```python
from build123d import *

# Parameters (mm, degrees)
F1_DEPTH = 7.5


with BuildPart() as f1:
    # F0 (on Top) → F1 (new body)
    with BuildSketch(Plane.XY):
        with BuildLine():
            ThreePointArc((0, 2), (0.585786, 0.585786), (2, 0))
            Line((2, 0), (8, 0))
            ThreePointArc((8, 0), (9.414214, 0.585786), (10, 2))
            Line((10, 2), (10, 45))
            ThreePointArc((10, 45), (9.414214, 46.414214), (8, 47))
            Line((8, 47), (-8.8, 47))
            ThreePointArc((-8.8, 47), (-10.214214, 46.414214), (-10.8, 45))
            Line((-10.8, 45), (-10.8, 39))
            ThreePointArc((-10.8, 39), (-10.214214, 37.585786), (-8.8, 37))
            Line((-8.8, 37), (-7.8, 37))
            ThreePointArc((-7.8, 37), (-6.385786, 37.585786), (-5.8, 39))
            Line((-5.8, 39), (-5.8, 42))
            Line((-5.8, 42), (0, 42))
            Line((0, 42), (0, 2))
        make_face()
    extrude(amount=F1_DEPTH)


solid = f1.part
```
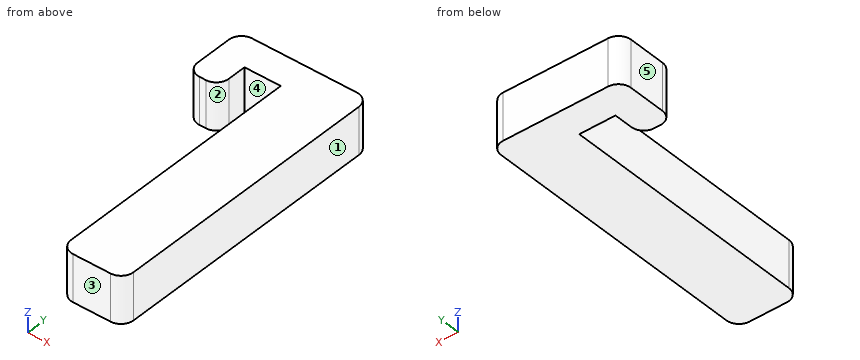
Geometry check sheet. Reference: the model listing, model coordinates, mm. Face numbers are marked on the shaded views. A direction names the side the tool comes from. Give positions to 0.01 mm unless a question says otherwise; leave off trailing zeros. Write each loop counter-clockwise with the first axis right and the second up, starting at its lowest first coordinate (ties: lowest second). Pieces come first, ordered by that corner, then holes. Notation, with made-up numbers: (-27.5, 36) - (17.5, 36) arc R30 ccw to (17.5, 67) - close; hole circle Ø7 at (54, -4.75). An arc over 180 degrees is marked (long way). Use a Markdown table: item, result.
Q1. Section check C-C, the plane x = -0.5. Enter the section's corners in (y, z).
Computed:
| item | result |
|---|---|
| outline | (42, 0) - (47, 0) - (47, 7.5) - (42, 7.5) - close |
Q2. Section check D-D, the plane y = 19. Enter the section's corners in (x, z).
Computed:
| item | result |
|---|---|
| outline | (0, 0) - (10, 0) - (10, 7.5) - (0, 7.5) - close |
Q3. Section check A-A, the plane y = 41. Enter the section's corners in (x, z), then the cut area to 4 significant figures.
Computed:
| item | result |
|---|---|
| outline | (-10.8, 0) - (-5.8, 0) - (-5.8, 7.5) - (-10.8, 7.5) - close; (0, 0) - (10, 0) - (10, 7.5) - (0, 7.5) - close |
| area | 112.5 mm² |
Q4. Set-up check for the marked faces 4 and 5: record each of +Z, -Z, +X, -X, +Y, -Y from which the full face is reachable in a straight line by a thin tool's end or side.
Computed:
| item | result |
|---|---|
| face 4 | +Z, -Z, -Y |
| face 5 | +Z, -Z, -X, +Y, -Y |
Q5. Thickness scan on L1, parallel to X at y = 19.5, z = 7; L2, parallel to Y at x = -8.5, z = 2; L3, parallel to Y at x = 0.25, z = 2.5. Record the ranges inside material, lowest first. Write a range as [from, to].
Computed:
| item | result |
|---|---|
| L1 | x = [0, 10] |
| L2 | y = [37, 47] |
| L3 | y = [1.03, 47] |
Q6. Draft check along X on the marked faces 1, 2 and 3. Enter one of: pulls with the +X half, pulls with the -X half, needs draft (parallel to the pull), parting line crosses it, or undercut.
Computed:
| item | result |
|---|---|
| face 1 | pulls with the +X half |
| face 2 | undercut |
| face 3 | needs draft |
Q7. Section check B-B, the plane z = 1.75. Enter the section's corners in (x, y), then the cut area to 3 significant figures.
Computed:
| item | result |
|---|---|
| outline | (-10.8, 39) arc R2 ccw to (-8.8, 37) - (-7.8, 37) arc R2 ccw to (-5.8, 39) - (-5.8, 42) - (0, 42) - (0, 2) arc R2 ccw to (2, 0) - (8, 0) arc R2 ccw to (10, 2) - (10, 45) arc R2 ccw to (8, 47) - (-8.8, 47) arc R2 ccw to (-10.8, 45) - close |
| area | 544 mm² |
